```python
from build123d import *

# Parameters (mm, degrees)
F0_R        = 1.45
F0_W        = 20
F0_H        = 11
F0_W_2      = 16
F0_H_2      = 8
F1_DEPTH    = 4
F2_DEPTH    = 10
F3_R        = 1.45
F4_DEPTH    = 25
F3_R_2      = 2.05
F5_DEPTH    = 11
F0_W_3      = 5
F0_H_3      = 7
F6_DEPTH    = 25
F7_T1_DEPTH = 31.5734639037
F7_T3_DEPTH = 24.5734639037
F8_R        = 1


# Not quite as in the source:
# - a fillet or chamfer that OpenCascade refuses, or shapes differently, is made with other operations: its cross-section is extruded or revolved along the edge and cut away or added


with BuildPart() as f1:
    # F0 (on Top) → F1 (new body)
    with BuildSketch(Plane.XY):
        with BuildLine():
            ThreePointArc((-28.4361224622, 2.6766185844), (-27.3113181327, 1.54304563), (-26.9, 0))
            ThreePointArc((-26.9, 0), (-27.3113181327, -1.54304563), (-28.4361224622, -2.6766185844))
            Line((-28.4361224622, -2.6766185844), (-28.4361224622, -5.5))
            Line((-28.4361224622, -5.5), (-3.3, -5.5))
            Line((-3.3, -5.5), (-3.3, 5.5))
            Line((-3.3, 5.5), (-28.4361224622, 5.5))
            Line((-28.4361224622, 5.5), (-28.4361224622, 2.6766185844))
        make_face()
        with Locations((-22, 0)):
            Circle(F0_R, mode=Mode.SUBTRACT)
        with BuildLine():
            Line((28.4361224622, 5.5), (16.7, 5.5))
            Line((16.7, 5.5), (16.7, -5.5))
            Line((16.7, -5.5), (28.4361224622, -5.5))
            Line((28.4361224622, -5.5), (28.4361224622, -2.6766185844))
            ThreePointArc((28.4361224622, -2.6766185844), (26.9, 0), (28.4361224622, 2.6766185844))
            Line((28.4361224622, 2.6766185844), (28.4361224622, 5.5))
        make_face()
        with Locations((22, 0)):
            Circle(F0_R, mode=Mode.SUBTRACT)
        with Locations((6.7, 0)):
            Rectangle(F0_W, F0_H)
        with Locations((6.7, 0)):
            Rectangle(F0_W_2, F0_H_2, mode=Mode.SUBTRACT)
    extrude(amount=-F1_DEPTH)

    # F0 (on Top) → F2 (join)
    with BuildSketch(Plane.XY):
        with Locations((6.7, 0)):
            Rectangle(F0_W, F0_H)
        with Locations((6.7, 0)):
            Rectangle(F0_W_2, F0_H_2, mode=Mode.SUBTRACT)
    extrude(amount=F2_DEPTH)

    # F3 (on face) → F4 (cut)
    with BuildSketch(Plane.XZ.offset(5.5)):
        with Locations((6.7, 6)):
            Circle(F3_R)
    extrude(amount=-F4_DEPTH, mode=Mode.SUBTRACT)

    # F3 (on face) → F5 (join, through all)
    with BuildSketch(Plane.XZ.offset(5.5)):
        with Locations((6.7, 6)):
            Circle(F3_R_2)
        with Locations((6.7, 6)):
            Circle(F3_R, mode=Mode.SUBTRACT)
    extrude(amount=-F5_DEPTH)

    # F0 (on Top) → F6 (cut)
    with BuildSketch(Plane.XY):
        with Locations((6.7, 0)):
            Rectangle(F0_W_3, F0_H_3)
    extrude(amount=F6_DEPTH, mode=Mode.SUBTRACT)

    # F7: chamfer of 4 on 6 edges, made by hand

    # F7_s2 → F7_t1 (cut)
    with BuildSketch(Plane.XZ.offset(-15.7867319519)):
        Polygon((-3.3, 6), (0.7, 10), (-3.3, 10), align=None)
        Polygon((12.7, 10), (16.7, 6), (16.7, 10), align=None)
    extrude(amount=F7_T1_DEPTH, mode=Mode.SUBTRACT)

    # F7_s4 → F7_t3 (cut)
    with BuildSketch(Plane.XY.offset(-14.2867319519)):
        Polygon((-28.4361224622, -1.5), (-24.4361224622, -5.5), (-28.4361224622, -5.5), align=None)
        Polygon((-28.4361224622, 1.5), (-24.4361224622, 5.5), (-28.4361224622, 5.5), align=None)
        Polygon((24.4361224622, -5.5), (28.4361224622, -1.5), (28.4361224622, -5.5), align=None)
        Polygon((24.4361224622, 5.5), (28.4361224622, 1.5), (28.4361224622, 5.5), align=None)
    extrude(amount=F7_T3_DEPTH, mode=Mode.SUBTRACT)

    # F8
    f8_edges = [f1.edges().sort_by_distance(p)[0] for p in [
        (-1.3, 0, 8),
        (14.7, 0, 8),
        (0.7, 4.75, 10),
        (0.7, -4.75, 10),
        (12.7, -4.75, 10),
        (12.7, 4.75, 10),
        (-3.3, 0, 0),
        (16.7, 0, 0),
    ]]
    fillet(f8_edges, radius=F8_R)


solid = f1.part
```
Check sheet for the modelled part. Datum: model origin and axes. Units: mm. A direction names the side the tool comes from. Give positions to 0.01 mm unless a question says otherwise; leave off trailing zeros. Write each loop counter-clockwise with the first axis right and the second up, starting at its lowest first coordinate (ties: lowest second). Pieces come first, ordered by that corner, then holes.
Item 1: Cross-section at B-B (z = 8.75). Enter the section's corners in (x, y), and give its area (3 significant figures).
Item 2: Scan lines: L1, parallel to Y at x = 6, z = 4.25; L2, parallel to Y at x = -22, z = -3.05; L3, parallel to Z at x = 6.7, y = -4.15. Record each from-to range of solid material in increasing order.
Item 3: Cross-section at C-C (z = 2.5). Enter the section's corners in (x, y), and give its area (3 significant figures).
Item 4: Access from +Z, -Z, +X, -X, +Y, -Y to the whole of each face (thin tool, end or side, straight path). Record for faces 1 (the face through (24, 0, 0)), 2 (the face through (15.333, 0.056, 6.516)), 3 (the face through (6.256, -3.754, 3.999)), 4 (the face through (-16, 0, 0)), 5 (the face through (-1.3, 0, 1)).
Item 5: Draft check along X on faces 6 (the face through (26.083, -3.853, -2.028)), 7 (the face through (7, -5, 10)), 8 (the face through (-26.13, -3.807, -2.028)), 9 (the face through (5, 3.5, 6)). Enter one of: released by +X, released by -X, zero draft, split by the parting line, or undercut.
Item 6: Cross-section at D-D (y = -4.5). Enter the section's corners in (x, z).
Item 7: Gauge pin test, flat ends, axial feed: pin 1 (3.5 mm diameter, centred on x = 22, y = 0, fed in from +Z); pin 2 (2 mm diameter, centred on y = 3.5, z = -2.5, fed in from -X); pin 3 (1 mm diameter, centred on y = 4, z = 0, fed in from -X). Record the tip position at first contact, or that the pin passes through.
Item 8: Cross-section at A-A (x = 22). Enter the section's corners in (y, z).
Report:
1. outline: (-0.55, -5.5) - (13.95, -5.5) - (13.95, -4) - (-0.55, -4) - close; (-0.55, 4) - (13.95, 4) - (13.95, 5.5) - (-0.55, 5.5) - close
1. area: 43.5 mm2
2. L1: y = -5.5 to -3.5, 3.5 to 5.5
2. L2: y = -5.5 to -1.45, 1.45 to 5.5
2. L3: z = -4 to 4.55, 7.45 to 10
3. outline: (-3.3, -5.5) - (16.7, -5.5) - (16.7, 5.5) - (-3.3, 5.5) - close; hole (-1.3, -4) - (14.7, -4) - (14.7, 4) - (-1.3, 4) - close
3. area: 92.0 mm2
4. face 1: +Z, +X, +Y, -Y
4. face 2: +Z
4. face 3: none
4. face 4: +Z, -X, +Y, -Y
4. face 5: +Z, -Z
5. face 6: released by +X
5. face 7: zero draft
5. face 8: released by -X
5. face 9: undercut
6. outline: (-25.44, -4) - (25.44, -4) - (25.44, 0) - (17.7, 0) arc R1 cw to (16.7, 1) - (16.7, 6) - (12.99, 9.71) arc R1 ccw to (12.29, 10) - (1.11, 10) arc R1 ccw to (0.41, 9.71) - (-3.3, 6) - (-3.3, 1) arc R1 cw to (-4.3, 0) - (-25.44, 0) - close; hole circle Ø2.9 at (6.7, 6)
7. pin 1: stops at z = 0
7. pin 2: stops at x = -27.44
7. pin 3: stops at x = -26.44
8. outline: (-5.5, -4) - (-1.45, -4) - (-1.45, 0) - (-5.5, 0) - close; (1.45, -4) - (5.5, -4) - (5.5, 0) - (1.45, 0) - close
